For this review, take the finished solid that the model builds, in its own axes (mm). Face numbers are marked on the shaded views. A direction names the side the tool comes from. Round coordinates to 2 decimals unless told otherwise and drop trailing zeros. Write each loop counter-clockwise with the first axis right and the second up, starting at its lowest first coordinate (ties: lowest second). Pieces come first, ordered by that corner, then holes. Notation, with made-up numbers: M 74.5,65 L 108.5,65 A30 cw 108.5,93 Z; hole C 70,-22.75 d10. An arc over 180 degrees is marked long. Use one line per item in the form item = value. Start each with the question number.
Item 1: Add section A-A (x = 0). State the section outline as (y, z) points.
Item 2: Add section B-B (x = -17). State the section outline as (y, z) points.
Item 3: For line 1 (Y direction, x = -17.5, z = 0.45); line 2 (Z direction, x = -1, y = -0.5); line 3 (Z direction, x = -1.5, y = 9), list the stretches that pass through material, from the lowest coordinate up. Write a range as [from, to].
Item 4: For the marked faces 1, 2, 3, 4 and 5, list the 3-axis set-ups (+Z, -Z, +X, -X, +Y, -Y) from which the entire face can be reached by the end or side of a thin tool; tool diameter is ignored.
Item 5: Add section D-D (y = -13). State the section outline as (x, z) points.
Item 6: For P1, Ø2.5, axis at y = -14.5, z = 14, coming from the +X side; P2, Ø2.5, axis at x = 17.5, y = 0, coming from the -Z side; P3, Ø5, axis at x = 9.5, y = 0, coming from the -Z side; P4, Ø0.8, axis at x = 15.5, z = 1, coming from the +Y side, all flat-tipped, find the tip position at first contact; note any pin that passes through.
Item 7: Add section C-C (z = 11). State the section outline as (x, y) points.
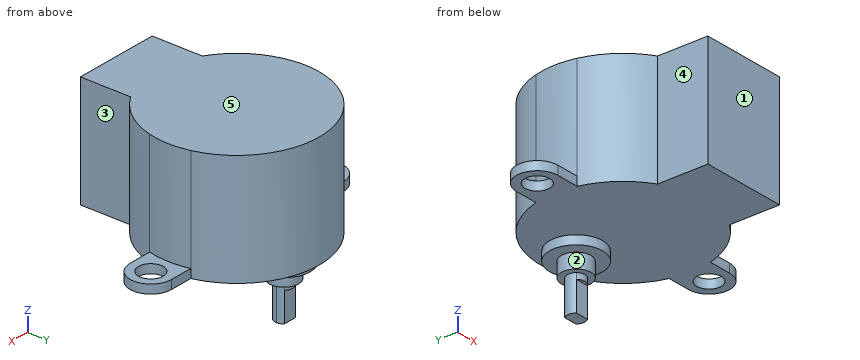
from build123d import *

# Parameters (mm, degrees)
F0_R          = 4.5
F1_DEPTH      = 19
F0_R_2        = 2.1
F2_DEPTH      = 1.5
F0_R_3        = 2.5
F3_DEPTH      = 1.5
F3_DEPTH_BACK = 19
F4_DEPTH      = 4
F4_DEPTH_BACK = 19
F5_DEPTH      = 10
F5_DEPTH_BACK = 19
F6_DEPTH      = 19
F6_DEPTH_BACK = 5


with BuildPart() as f1:
    # F0 (on Top) → F1 (new body)
    with BuildSketch(Plane.XY):
        with BuildLine():
            ThreePointArc((13.5554417117, 3.5), (0, 14), (-13.5554417117, 3.5))
            ThreePointArc((-13.5554417117, 3.5), (-14, 0), (-13.5554417117, -3.5))
            ThreePointArc((-13.5554417117, -3.5), (-11.250406053, -8.3323684294), (-7.3, -11.9461290802))
            Line((-7.3, -11.9461290802), (-7.3, -20.5))
            Line((-7.3, -20.5), (7.3, -20.5))
            Line((7.3, -20.5), (7.3, -11.9461290802))
            ThreePointArc((7.3, -11.9461290802), (11.250406053, -8.3323684294), (13.5554417117, -3.5))
            ThreePointArc((13.5554417117, -3.5), (14, 0), (13.5554417117, 3.5))
        make_face()
        with Locations((0, 8)):
            Circle(F0_R, mode=Mode.SUBTRACT)
    extrude(amount=F1_DEPTH)

    # F0 (on Top) → F2 (join)
    with BuildSketch(Plane.XY):
        with BuildLine():
            Line((-13.5554417117, 3.5), (-17.5, 3.5))
            ThreePointArc((-17.5, 3.5), (-21, 0), (-17.5, -3.5))
            Line((-17.5, -3.5), (-13.5554417117, -3.5))
            ThreePointArc((-13.5554417117, -3.5), (-14, 0), (-13.5554417117, 3.5))
        make_face()
        with Locations((-17.5, 0)):
            Circle(F0_R_2, mode=Mode.SUBTRACT)
        with BuildLine():
            Line((17.5, 3.5), (13.5554417117, 3.5))
            ThreePointArc((13.5554417117, 3.5), (14, 0), (13.5554417117, -3.5))
            Line((13.5554417117, -3.5), (17.5, -3.5))
            ThreePointArc((17.5, -3.5), (21, 0), (17.5, 3.5))
        make_face()
        with Locations((17.5, 0)):
            Circle(F0_R_2, mode=Mode.SUBTRACT)
    extrude(amount=F2_DEPTH)

    # F0 (on Top) → F3 (join, two sides)
    with BuildSketch(Plane.XY) as f3_sk:
        with Locations((0, 8)):
            Circle(F0_R)
        with Locations((0, 8)):
            Circle(F0_R_3, mode=Mode.SUBTRACT)
    extrude(amount=-F3_DEPTH)
    extrude(f3_sk.sketch, amount=F3_DEPTH_BACK)

    # F0 (on Top) → F4 (join, two sides)
    with BuildSketch(Plane.XY) as f4_sk:
        with Locations((0, 8)):
            Circle(F0_R_3)
        with BuildLine():
            ThreePointArc((1.1180339887, 9), (1.4012585384, 8.5352331347), (1.5, 8))
            ThreePointArc((1.5, 8), (1.4012585384, 7.4647668653), (1.1180339887, 7))
            ThreePointArc((1.1180339887, 7), (0, 6.5), (-1.1180339887, 7))
            ThreePointArc((-1.1180339887, 7), (-1.5, 8), (-1.1180339887, 9))
            ThreePointArc((-1.1180339887, 9), (0, 9.5), (1.1180339887, 9))
        make_face(mode=Mode.SUBTRACT)
    extrude(amount=-F4_DEPTH)
    extrude(f4_sk.sketch, amount=F4_DEPTH_BACK)

    # F0 (on Top) → F5 (join, two sides)
    with BuildSketch(Plane.XY) as f5_sk:
        with BuildLine():
            ThreePointArc((1.1180339887, 7), (1.4012585384, 7.4647668653), (1.5, 8))
            ThreePointArc((1.5, 8), (1.4012585384, 8.5352331347), (1.1180339887, 9))
            Line((1.1180339887, 9), (-1.1180339887, 9))
            ThreePointArc((-1.1180339887, 9), (-1.5, 8), (-1.1180339887, 7))
            Line((-1.1180339887, 7), (1.1180339887, 7))
        make_face()
    extrude(amount=-F5_DEPTH)
    extrude(f5_sk.sketch, amount=F5_DEPTH_BACK)

    # F0 (on Top) → F6 (join, two sides)
    with BuildSketch(Plane.XY) as f6_sk:
        with BuildLine():
            ThreePointArc((-1.1180339887, 7), (0, 6.5), (1.1180339887, 7))
            Line((1.1180339887, 7), (-1.1180339887, 7))
        make_face()
        with BuildLine():
            Line((-1.1180339887, 9), (1.1180339887, 9))
            ThreePointArc((1.1180339887, 9), (0, 9.5), (-1.1180339887, 9))
        make_face()
    extrude(amount=F6_DEPTH)
    extrude(f6_sk.sketch, amount=-F6_DEPTH_BACK)


solid = f1.part
Calculated:
q1.outline = M -20.5,0 L 3.5,0 L 3.5,-1.5 L 5.5,-1.5 L 5.5,-4 L 6.5,-4 L 6.5,-5 L 7,-5 L 7,-10 L 9,-10 L 9,-5 L 9.5,-5 L 9.5,-4 L 10.5,-4 L 10.5,-1.5 L 12.5,-1.5 L 12.5,0 L 14,0 L 14,19 L -20.5,19 Z
q2.outline = M -3.5,0 L -2.04,0 L -2.04,1.5 L -3.5,1.5 Z; M 2.04,0 L 3.5,0 L 3.5,1.5 L 2.04,1.5 Z
q3.line_1 = [-3.5, -2.1], [2.1, 3.5]
q3.line_2 = [0, 19]
q3.line_3 = [-4, 19]
q4.face_1 = +Z, -Z, +X, -X, -Y
q4.face_2 = -Z
q4.face_3 = +Z, -Z, +X, -Y
q4.face_4 = +Z, -Z, -X, -Y
q4.face_5 = +Z, +X, -X, +Y, -Y
q5.outline = M -7.3,0 L 7.3,0 L 7.3,19 L -7.3,19 Z
q6.P1 = 7.3
q6.P2 = through
q6.P3 = 0
q6.P4 = 3.5
q7.outline = M -7.3,-20.5 L 7.3,-20.5 L 7.3,-11.95 A14 ccw long -7.3,-11.95 Z
